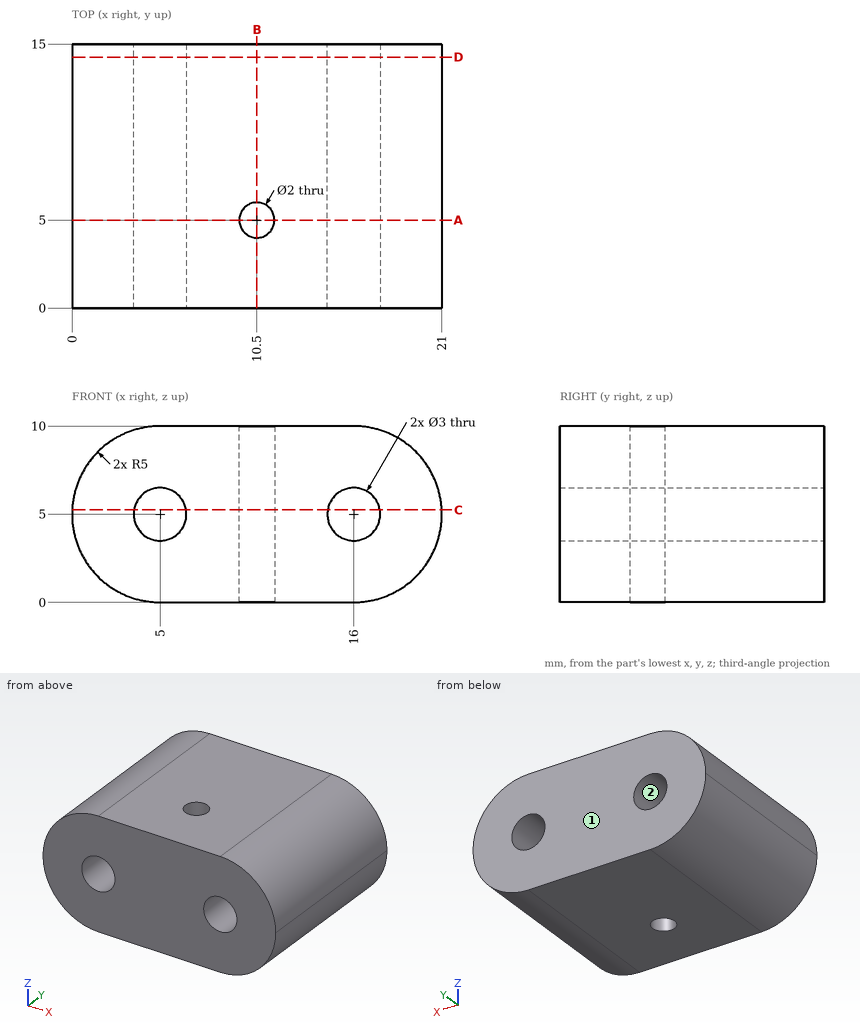
Check sheet for the drawn part. Datum: minimum x, y, z corner. Units: mm. Round coordinates to 2 decimals unless told otherwise and drop trailing zeros. Loops run counter-clockwise (first coordinate to the right, second up) from the corner with the lowest first, then second, coordinate; pieces in that order, holes last. Notation, with made-up numbers: (-18.75, 13) -> (-2.75, 13) arc R36 cw to (-2.75, 47) -> close; hole circle Ø1 at (40.25, 87.5). An arc over 180 degrees is marked (long way). Put each result on its own line as item: value. Start each with the question number.
1. Section check A-A (y = 5). Enter the section's corners in (x, z), plus the area to 3 significant figures.
2. Section check C-C (z = 5.25). Enter the section's corners in (x, y), plus the area to 3 significant figures.
3. Scan lines: probe 1 along Y at (x, z) = (10.5, 7.5); probe 2 along Z at (x, y) = (5, 5.5); probe 3 along Y at (x, z) = (9.75, 8.25). Record each from-to range of solid material in increasing order.
4. Section check B-B (x = 10.5). Enter the section's corners in (y, z), plus the area to 3 significant figures.
5. Gauge pin test, flat end, axial feed: pin 1 (5 mm diameter, centred on x = 3, y = 10, fed in from +Z). Record the tip position at first contact, or that the pin passes through.
6. Draft check along X on the marked faces 1 and 2. Enter one of: +X half, -X half, draft (parallel to the pull), parting line (faces both ways), or undercut.
7. Section check D-D (y = 14.25). Enter the section's corners in (x, z).
Findings:
1. outline: (5, 0) -> (9.5, 0) -> (9.5, 10) -> (5, 10) arc R5 ccw to start; (11.5, 0) -> (16, 0) arc R5 ccw to (16, 10) -> (11.5, 10) -> close; hole circle Ø3 at (5, 5); hole circle Ø3 at (16, 5)
1. area: 154 mm^2
2. outline: (0.01, 0) -> (3.52, 0) -> (3.52, 15) -> (0.01, 15) -> close; (6.48, 0) -> (14.52, 0) -> (14.52, 15) -> (6.48, 15) -> close; (17.48, 0) -> (20.99, 0) -> (20.99, 15) -> (17.48, 15) -> close; hole circle Ø2 at (10.5, 5)
2. area: 223 mm^2
3. probe 1: y = 0 to 4, 6 to 15
3. probe 2: z = 0 to 3.5, 6.5 to 10
3. probe 3: y = 0 to 4.34, 5.66 to 15
4. outline: (0, 0) -> (4, 0) -> (4, 10) -> (0, 10) -> close; (6, 0) -> (15, 0) -> (15, 10) -> (6, 10) -> close
4. area: 130 mm^2
5. pin 1: stops at z = 10
6. face 1: draft
6. face 2: undercut
7. outline: (5, 0) -> (16, 0) arc R5 ccw to (16, 10) -> (5, 10) arc R5 ccw to start; hole circle Ø3 at (5, 5); hole circle Ø3 at (16, 5)
